For this review, take the finished solid that the model builds, in its own axes (mm). Round coordinates to 2 decimals unless told otherwise and drop trailing zeros. Order: outer loops, then holes, each group sorted by start corner. A loop starts at its lowest first (then second) coordinate and runs counter-clockwise, first axis right, second up. Notation, with made-up numbers: M 66.5,17 L 85.5,17 A29 ccw 85.5,52 Z; hole C 85.5,-29 d4. An arc over 180 degrees is marked long. Put each result on its own line as item: value.
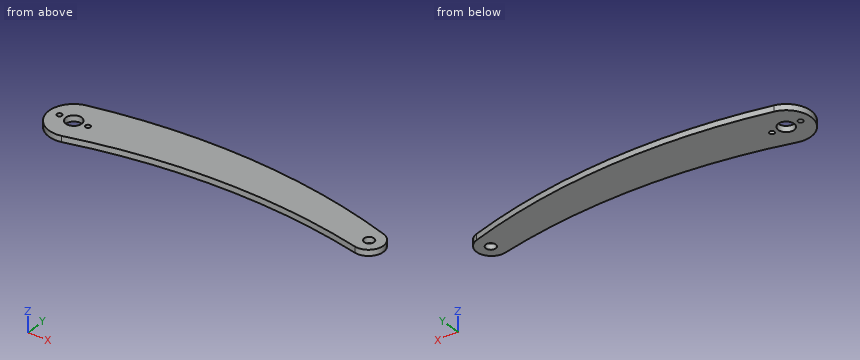
Autodesk Inventor part; units mm, degrees
ref_plane "YZ Plane" through (0, 0, 0) normal (1, 0, 0) x (0, 1, 0)
ref_plane "XZ Plane" through (0, 0, 0) normal (0, 1, 0) x (-1, 0, 0)
ref_plane "XY Plane" through (0, 0, 0) normal (0, 0, 1) x (1, 0, 0)
sketch "Sketch1" plane through (0, 0, 0) normal (0, 0, 1) x (1, 0, 0)
  line L0 (0, 0) -> (150, 0) construction
  circle A0 centre (0, 0) radius 4
  circle A1 centre (0, 0) radius 12.5 construction
  circle A2 centre (150, 0) radius 2.5
  circle A3 centre (150, 0) radius 7.5 construction
  arc A4 (150, 0) -> (0, 0) centre (75, -290.4738) ccw construction
  line L1 (-4.0971, 17.3539) -> (0, 0) construction
  line L2 (0, 0) -> (12.1656, 2.8722) construction
  line L3 (0, 0) -> (3.4621, -14.6644) construction
  line L4 (147.6861, -9.448) -> (150, 0) construction
  line L5 (150, 0) -> (152.7079, 11.057) construction
  line L6 (150, 0) -> (150, 0) construction
  line L7 (150, 0) -> (142.7153, 1.7841) construction
  arc A5 (151.7841, 7.2847) -> (-2.8722, 12.1656) centre (65.313, -279.983) ccw
  arc A6 (148.2159, -7.2847) -> (2.8722, -12.1656) centre (85.3125, -300.6159) ccw
  arc A7 (-2.8722, 12.1656) -> (2.8722, -12.1656) centre (-0.0311, -0.0073) ccw
  arc A8 (148.2159, -7.2847) -> (151.7841, 7.2847) centre (149.6194, 0.0932) ccw
  circle A9 centre (-0.0311, -0.0073) radius 7.25 construction
  circle A10 centre (-7.2811, 0) radius 1.25
  circle A11 centre (7.2189, 0) radius 1.25
  dimension "d0" = 150
  dimension "d1" = 8
  dimension "d2" = 25
  dimension "d3" = 5
  dimension "d4" = 15
  dimension "d6" = 300
  dimension "d7" = 90
  dimension "d8" = 180
  dimension "d9" = 180
  dimension "d10" = 90
  dimension "d11" = 300
  dimension "d12" = 300
  dimension "d13" = 14.5
  dimension "d14" = 2.5
  dimension "d15" = 2.5
extrude "Extrusion1" add sketch "Sketch1" along normal blind 3
properties part number "brazo"
(1) To check wall thickness, follow L1, parallel to X at y = -0.5, z = 2.25; L2, parallel to X at y = 2, z = 2.35; L3, parallel to Y at x = 0, z = 2. State the ranges of each line that lie inside material, in increasing order.
A:
L1: x = -12.52 to -8.43, -6.14 to -3.97, 3.97 to 6.07, 8.36 to 147.55, 152.45 to 157.11
L2: x = -12.37 to -3.46, 3.46 to 148.5, 151.5 to 156.88
L3: y = -12.51 to -4, 4 to 12.82
(2) Add section C-C on x = 0. Give the boundary of the cut face in (y, z), then the cut area to 3 significant figures.
A:
outline: M -12.51,0 L -4,0 L -4,3 L -12.51,3 Z; M 4,0 L 12.82,0 L 12.82,3 L 4,3 Z
area: 52.0 mm2
(3) Add section A-A on x = 150. Give the boundary of the cut face in (y, z).
A:
outline: M -7.41,0 L -2.5,0 L -2.5,3 L -7.41,3 Z; M 2.5,0 L 7.82,0 L 7.82,3 L 2.5,3 Z
(4) Add section B-B on z = 0.85. Give the boundary of the cut face in (x, y), then the cut area to 3 significant figures.
A:
outline: M -2.87,12.17 A12.5 ccw 2.87,-12.17 A300 cw 148.22,-7.28 A7.51 ccw 151.78,7.28 A300 ccw Z; hole C -7.28,0 d2.5; hole C 0,0 d8; hole C 7.22,0 d2.5; hole C 150,0 d5
area: 3,350 mm2
(5) Insertion check: pin 1 Ø7 at (x, y) = (0, 0) entering from -Z; pin 2 Ø1 at (x, z) = (105, 2.5) entering from -Y; pin 3 Ø1.5 at (x, z) = (83.5, 2) entering from +Y. Each pin has a flat end and moves straight along its axis. Give the tip position at first contact, or say it passes through.
A:
pin 1: passes through
pin 2: stops at y = -1.3
pin 3: stops at y = 19.51
